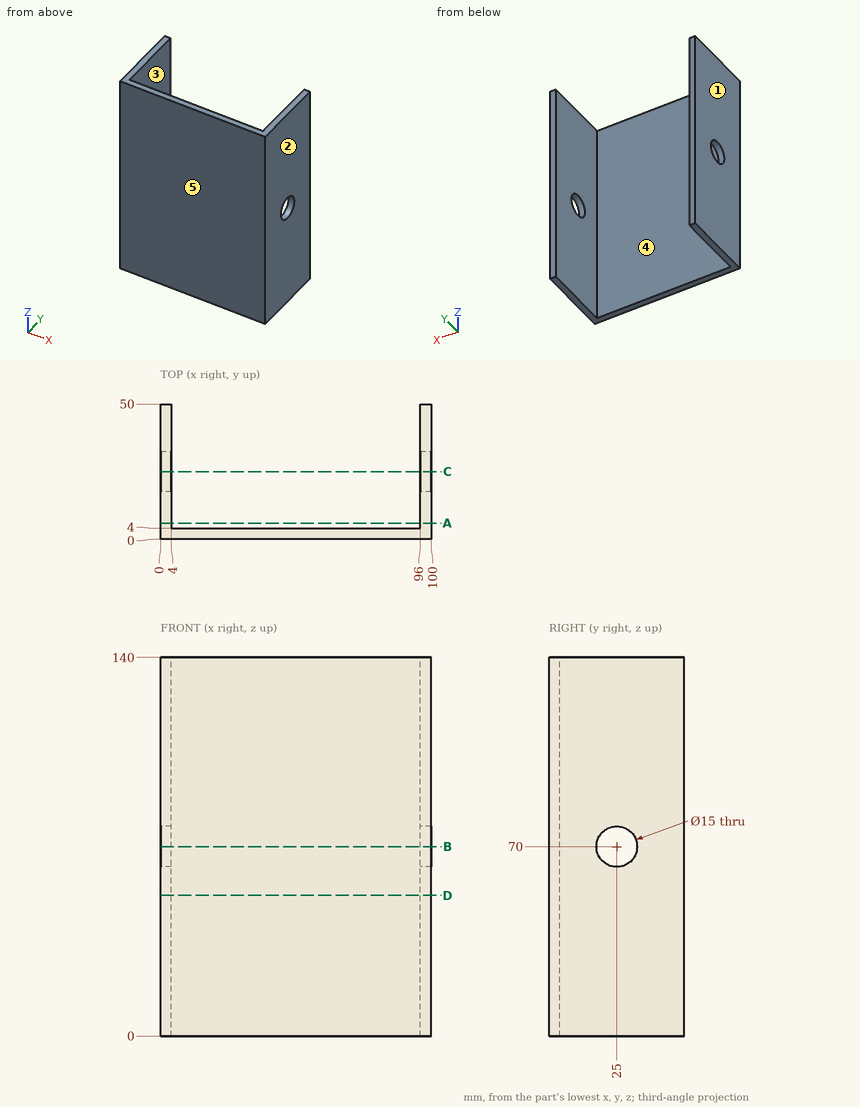
Study the drawing (mm; zero at the part's minimum x, y, z) and answer. A direction names the side the tool comes from. Give positions to 0.01 mm unless a question says otherwise; leave off trailing zeros. Write each loop counter-clockwise with the first axis right and the second up, starting at its lowest first coordinate (ties: lowest second). Pieces come first, ordered by that corner, then holes. Notation, with made-up numbers: (14.5, -2) -> (24.5, -2) arc R32 ccw to (24.5, 26) -> close; hole circle Ø4 at (49.25, 18.25). An arc over 180 degrees is marked (long way). Answer as a JSON object with one key per item and string values. Group by question number.
1) A tool of negligible diameter and unlimited length cuts with its end or side. For the marked faces 4 and 5, from which of +Z, -Z, +X, -X, +Y, -Y can it reach the whole face along a straight path? Write none if from no direction.
2) Find section B-B (z = 70). Write down the section's boundary in (x, y), and give its area (3 significant figures).
3) The mould has two halves that part along X. Classify the marked faces 1, 2 and 3: +X half, -X half, draft (parallel to the pull), parting line (faces both ways), or undercut.
4) Consider L1, parallel to X at y = 14, z = 125; L2, parallel to Z at x = 1.05, y = 25; L3, parallel to Y at x = 2.25, z = 70. Determine where each line is inside the solid, lowest interval first. Write a range as from..to.
5) Find section A-A (y = 6). Write down the section's boundary in (x, z), and give its area (3 significant figures).
6) Find section D-D (z = 52). Write down the section's boundary in (x, y), and give its area (3 significant figures).
7) This flat-tipped pin is pushed along its axis until it touches: P1, Ø12, axis at x = 17.5, z = 121, coming from the +Y side. Where does it stop, or does it pass through?
8) Find section C-C (y = 25). Write down the section's boundary in (x, z), and give its area (3 significant figures).
Values follow:
{
 "1": {"face 4": "+Z, -Z, +Y", "face 5": "+Z, -Z, +X, -X, -Y"},
 "2": {"outline": "(0, 0) -> (100, 0) -> (100, 17.5) -> (96, 17.5) -> (96, 4) -> (4, 4) -> (4, 17.5) -> (0, 17.5) -> close; (0, 32.5) -> (4, 32.5) -> (4, 50) -> (0, 50) -> close; (96, 32.5) -> (100, 32.5) -> (100, 50) -> (96, 50) -> close", "area": "648 mm2"},
 "3": {"face 1": "-X half", "face 2": "+X half", "face 3": "undercut"},
 "4": {"L1": "x = 0..4, 96..100", "L2": "z = 0..62.5, 77.5..140", "L3": "y = 0..17.5, 32.5..50"},
 "5": {"outline": "(0, 0) -> (4, 0) -> (4, 140) -> (0, 140) -> close; (96, 0) -> (100, 0) -> (100, 140) -> (96, 140) -> close", "area": "1,120 mm2"},
 "6": {"outline": "(0, 0) -> (100, 0) -> (100, 50) -> (96, 50) -> (96, 4) -> (4, 4) -> (4, 50) -> (0, 50) -> close", "area": "768 mm2"},
 "7": {"P1": "stops at y = 4"},
 "8": {"outline": "(0, 0) -> (4, 0) -> (4, 62.5) -> (0, 62.5) -> close; (0, 77.5) -> (4, 77.5) -> (4, 140) -> (0, 140) -> close; (96, 0) -> (100, 0) -> (100, 62.5) -> (96, 62.5) -> close; (96, 77.5) -> (100, 77.5) -> (100, 140) -> (96, 140) -> close", "area": "1,000 mm2"}
}
